Build history of the part. All positions in model axes, mm. A direction names the side the tool comes from. Give positions to 0.01 mm unless a question says otherwise; leave off trailing zeros. Loops run counter-clockwise (first coordinate to the right, second up) from the corner with the lowest first, then second, coordinate; pieces in that order, holes last. Notation, with made-up numbers: (62.5, 14.25) - (114.5, 14.25) arc R19 cw to (114.5, 44.25) - close; hole circle Ø11 at (-25, -33). An arc over 180 degrees is marked (long way). Return JSON: item names as keys, results as strings. Group by question number.
1) Slice it at C-C (y = 12). List the corners of the cut face in (x, z), and give its area (3 significant figures).
2) Slice it at B-B (x = 17). List the corners of the cut face in (y, z), and give its area (3 significant figures).
3) Drill centre lines: probe 1 along Y at (x, z) = (-0.5, 17.5); probe 2 along Y at (x, z) = (-0.5, 37); probe 3 along Y at (x, z) = (21.5, -10.5). Where is each one in solid material? Low to high. Write a range as from..to.
4) Mould opens along Z. For faces 1 (the face through (20.015, 2, 0)), 2 (the face through (-23.876, 2, 0)), 3 (the face through (12, 2, 25.4)), 4 (the face through (0.042, 25.557, -30.295)) say: released by +Z, released by -Z, zero draft, split by the parting line, or undercut.
5) Slice it at A-A (z = 13.5). List the corners of the cut face in (x, y).
6) 3-axis set-ups, long thin cutter, end or side, ignore diameter. For faces 5 (the face through (-12, 2, -25.4)), 6 (the face through (-0.08, 15.04, 25.93)), 7 (the face through (16.711, 2.447, -21.665)), 8 (the face through (-12, 2, 25.4)), 9 (the face through (-13, 4.826, 0)): which of +Z, -Z, +X, -X, +Y, -Y reach the whole face in a straight line?
7) Drop flat-ended pins along their axis: pin 1 (0.9 mm diameter, centred on x = 1, z = -31, fed in from +Y); pin 2 (4 mm diameter, centred on x = -10, y = 3.5, fed in from +Z); pin 3 (2 mm diameter, centred on x = 1, y = 19.5, fed in from -Z). Give the stop position or say it passes through.
Autodesk Inventor part; units mm, degrees
ref_plane "YZ Plane" through (0, 0, 0) normal (1, 0, 0) x (0, 1, 0)
ref_plane "XZ Plane" through (0, 0, 0) normal (0, 1, 0) x (-1, 0, 0)
ref_plane "XY Plane" through (0, 0, 0) normal (0, 0, 1) x (1, 0, 0)
sketch "Sketch1" plane through (0, 0, 0) normal (0, 1, 0) x (-1, 0, 0)
  line L0 (23.876, 25.4) -> (-23.876, 25.4)
  line L1 (23.876, -25.4) -> (23.876, 25.4)
  line L2 (-23.876, -25.4) -> (23.876, -25.4)
  line L3 (-23.876, 25.4) -> (-23.876, -25.4)
  point P0 (0, 0)
extrude "Extrusion1" add sketch "Sketch1" along normal blind 4.826
fillet "Fillet1" radius 5.842 4 edges at (23.876, 2.413, 25.4) (23.876, 2.413, -25.4) (-23.876, 2.413, 25.4) (-23.876, 2.413, -25.4)
sketch "Sketch2" plane through (0, 4.826, 0) normal (0, 1, 0) x (1, 0, 0)
  line L0 (-23.876, 19.558) -> (-23.876, -19.558)
  line L1 (23.876, -19.558) -> (23.876, 19.558)
  line L2 (18.034, 25.4) -> (-18.034, 25.4)
  line L3 (-20.0152, -18.288) -> (-20.0152, 18.288)
  arc A0 (-13.2588, 18.288) -> (-20.0152, 18.288) centre (-16.637, 18.288) ccw
  line L4 (-13.2588, 18.288) -> (-13.2588, -18.288)
  arc A1 (-20.0152, -18.288) -> (-13.2588, -18.288) centre (-16.637, -18.288) ccw
  line L5 (0, 26.1612) -> (0, 0) construction
  line L6 (20.0152, -18.288) -> (20.0152, 18.288)
  arc A2 (20.0152, 18.288) -> (13.2588, 18.288) centre (16.637, 18.288) ccw
  line L7 (13.2588, 18.288) -> (13.2588, -18.288)
  arc A3 (13.2588, -18.288) -> (20.0152, -18.288) centre (16.637, -18.288) ccw
  dimension "d3" = 3.3782
  dimension "d5" = 36.576
  dimension "d6" = 7.239
  dimension "d7" = 7.112
extrude "Extrusion2" cut sketch "Sketch2" against normal up to next
sketch "Sketch3" plane through (0, 0, 0) normal (1, 0, 0) x (0, 1, 0)
  line L0 (17.8879, 50.0199) -> (0, 28.702)
  line L1 (17.8879, 50.0199) -> (17.8879, 26.924)
  line L2 (14.097, 26.924) -> (17.8879, 26.924)
  line L3 (14.097, -12.7) -> (14.097, 26.924)
  line L4 (17.399, -39.4626) -> (17.399, -12.7)
  line L5 (14.097, -40.0449) -> (17.399, -39.4626)
  line L6 (0, -29.422) -> (14.097, -40.0449)
  line L7 (17.399, -12.7) -> (14.097, -12.7)
  line L8 (0, 28.702) -> (0, -29.422)
  point P0 (0, 0)
extrude "Extrusion3" add sketch "Sketch3" along normal mid plane 11.176
fillet "Fillet2" radius 3.302 2 edges at (0, 14.097, -12.7) (0, 14.097, 26.924)
sketch "Sketch4" plane through (0, 0, 0) normal (1, 0, 0) x (0, 1, 0)
  line L0 (17.399, -39.4626) -> (30.226, -37.2009)
  line L1 (30.226, -37.2009) -> (30.226, -25.0191)
  line L2 (30.226, -25.0191) -> (17.399, -22.0578)
  line L3 (17.399, -22.0578) -> (17.399, -39.4626)
  point P0 (0, 0)
extrude "Extrusion4" add sketch "Sketch4" along normal mid plane 6.0452
fillet "Fillet3" radius 5.588 2 edges at (0, 30.226, -25.0191) (0, 30.226, -37.2009)
sketch "Sketch6" plane through (0, 0, 0) normal (1, 0, 0) x (0, 1, 0)
  line L0 (33.401, 26.924) -> (30.226, 26.924)
  line L1 (33.401, 51.276) -> (31.226, 51.276)
  line L2 (33.401, 26.924) -> (33.401, 51.276)
  line L3 (30.226, 50.276) -> (31.226, 51.276)
  line L4 (24.638, 51.276) -> (24.638, 26.924) construction
  line L5 (17.8879, 50.0199) -> (17.8879, 26.924) construction
  line L6 (30.226, 26.924) -> (30.226, 50.276)
  point P0 (0, 0)
  dimension "d27" = 3.175
  dimension "d28" = 24.352
  dimension "d29" = 2.175
  dimension "d30" = 1
  dimension "d31" = 1
  dimension "d33" = 24.352
  dimension "d38" = 12.3381
  dimension "d40" = 4.6584
revolve "Revolution1" add sketch "Sketch6" angle 360 about axis through (0, 24.638, 51.276) along (0, 0, -1)
sketch "Sketch7" plane through (-3.0226, 0, 0) normal (-1, 0, 0) x (0, 0, 1)
  line L0 (-12.7, 17.399) -> (-39.4626, 17.399)
  point P0 (0, 0)
  point P1 (-32.512, 24.638)
  dimension "d42" = 7.239
  dimension "d43" = 6.9506
hole "Hole2" at (-3.0226, 24.638, -32.512) direction (1, 0, 0) diameter 4.8006 end through all
properties part number "Base_1"
Results:
{
 "1": {"outline": "(-5.59, -38.46) - (5.59, -38.46) - (5.59, 43) - (-5.59, 43) - close", "area": "910 mm2"},
 "2": {"outline": "(0, -25.4) - (4.83, -25.4) - (4.83, -21.65) - (0, -21.65) - close; (0, 21.65) - (4.83, 21.65) - (4.83, 25.4) - (0, 25.4) - close", "area": "36.2 mm2"},
 "3": {"probe 1": "0..14.1", "probe 2": "6.96..19.07, 30.2..33.39", "probe 3": "0..4.83"},
 "4": {"face 1": "undercut", "face 2": "zero draft", "face 3": "released by +Z", "face 4": "undercut"},
 "5": {"outline": "(-23.88, 0) - (-20.02, 0) - (-20.02, 4.83) - (-23.88, 4.83) - close; (-13.26, 0) - (13.26, 0) - (13.26, 4.83) - (5.59, 4.83) - (5.59, 14.1) - (-5.59, 14.1) - (-5.59, 4.83) - (-13.26, 4.83) - close; (20.02, 0) - (23.88, 0) - (23.88, 4.83) - (20.02, 4.83) - close"},
 "6": {"face 5": "-Z, -X, +Y, -Y", "face 6": "+X, -X, +Y", "face 7": "+Y, -Y", "face 8": "+Z, -X, +Y, -Y", "face 9": "+Z, -Z, -X, +Y"},
 "7": {"pin 1": "y = 30.23", "pin 2": "z = 25.4", "pin 3": "z = -39.27"}
}
